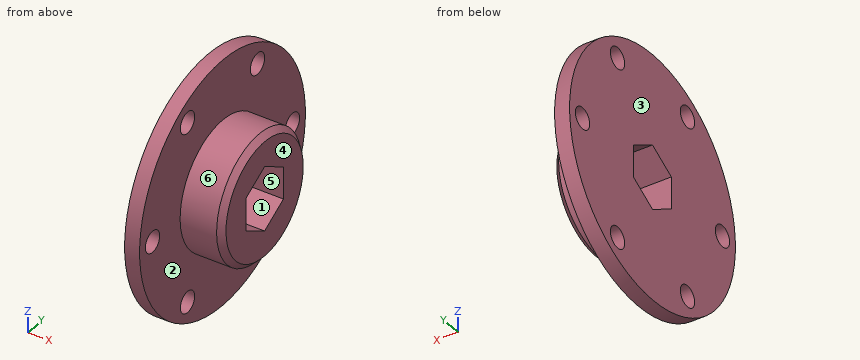
```python
from build123d import *

# Parameters (mm, degrees)
SKETCH1_R           = 27.94
SKETCH1_R_2         = 2.413
BOSS_EXTRUDE1_DEPTH = 3.3909
SKETCH2_R           = 14.2875
BOSS_EXTRUDE2_DEPTH = 9.525
CHAMFER1_SIZE       = 1.27


with BuildPart() as part:
    # Sketch1 → Boss-Extrude1 (new body)
    with BuildSketch(Plane(origin=(0, 0, 0), x_dir=(0, 0, -1), z_dir=(1, 0, 0))):
        Circle(SKETCH1_R)
        with Locations((0, 23.5839)):
            Circle(SKETCH1_R_2, mode=Mode.SUBTRACT)
        with Locations((20.42425652, 11.79195)):
            Circle(SKETCH1_R_2, mode=Mode.SUBTRACT)
        with Locations((20.42425652, -11.79195)):
            Circle(SKETCH1_R_2, mode=Mode.SUBTRACT)
        with Locations((0, -23.5839)):
            Circle(SKETCH1_R_2, mode=Mode.SUBTRACT)
        with Locations((-20.42425652, -11.79195)):
            Circle(SKETCH1_R_2, mode=Mode.SUBTRACT)
        with Locations((-20.42425652, 11.79195)):
            Circle(SKETCH1_R_2, mode=Mode.SUBTRACT)
        Polygon((7.332348419, 0), (3.666174209, 6.35), (-3.666174209, 6.35), (-7.332348419, 0), (-3.666174209, -6.35), (3.666174209, -6.35), align=None, mode=Mode.SUBTRACT)
    extrude(amount=BOSS_EXTRUDE1_DEPTH)

    # Sketch2 → Boss-Extrude2 (add)
    with BuildSketch(Plane(origin=(3.3909, 0, 0), x_dir=(0, 0, -1), z_dir=(1, 0, 0))):
        Circle(SKETCH2_R)
        Polygon((3.666174209, -6.35), (7.332348419, 0), (3.666174209, 6.35), (-3.666174209, 6.35), (-7.332348419, 0), (-3.666174209, -6.35), align=None, mode=Mode.SUBTRACT)
    extrude(amount=BOSS_EXTRUDE2_DEPTH)

    # Chamfer1
    chamfer1_edges = [part.edges().sort_by_distance(p)[0] for p in [
        (12.9159, 0, 14.2875),
    ]]
    chamfer(chamfer1_edges, length=CHAMFER1_SIZE)


solid = part.part
```
Work out the finished part from the listing and answer in its coordinate system (mm). Face numbers are marked on the shaded views. A direction names the side the tool comes from. Coordinates: 2 decimals unless noted, no trailing zeros. Order: outer loops, then holes, each group sorted by start corner. A loop starts at its lowest first (then second) coordinate and runs counter-clockwise, first axis right, second up. Notation, with made-up numbers: (75.5, 56.5) - (114.5, 56.5) arc R30 ccw to (114.5, 88.5) - close; hole circle Ø4 at (27.25, 41.5). An arc over 180 degrees is marked (long way). Answer as a JSON object with one key per item and string values.
1. Consider line 1 (Z direction, x = 2.75, y = -12.5); line 2 (Y direction, x = 3, z = -2); line 3 (X direction, y = 16, z = -7.5). Determine where each line is inside the solid, lowest interval first.
Output values:
{"line 1": "z = -24.99 to -22.73, -18.12 to 18.12, 22.73 to 24.99", "line 2": "y = -27.87 to -24.93, -22.23 to -6.35, 6.35 to 22.23, 24.93 to 27.87", "line 3": "x = 0 to 3.39"}
2. Find section A-A on z = 0. Determine the outline of the cut face in (x, y), plus the area to 3 significant figures.
Output values:
{"outline": "(0, -27.94) - (3.39, -27.94) - (3.39, -26) - (0, -26) - close; (0, -21.17) - (3.39, -21.17) - (3.39, -14.29) - (11.65, -14.29) - (12.92, -13.02) - (12.92, -6.35) - (0, -6.35) - close; (0, 6.35) - (12.92, 6.35) - (12.92, 13.02) - (11.65, 14.29) - (3.39, 14.29) - (3.39, 21.17) - (0, 21.17) - close; (0, 26) - (3.39, 26) - (3.39, 27.94) - (0, 27.94) - close", "area": "263 mm²"}
3. A tool of negligible diameter and unlimited length cuts with its end or side. For the marked faces 1, 2 and 3, from which of +Z, -Z, +X, -X, +Y, -Y can it reach the whole face along a straight path? Write none if from no direction.
Output values:
{"face 1": "+X, -X", "face 2": "+X", "face 3": "+Z, -Z, -X, +Y, -Y"}
4. The mould has two halves that part along Z. Classify the marked faces 4, 5 and 6: +Z half, -Z half, draft (parallel to the pull), parting line (faces both ways), or undercut.
Output values:
{"face 4": "draft", "face 5": "undercut", "face 6": "parting line"}
5. Each of these flat-tipped pins is pushed along its axis until it touches: P1, Ø2, axis at y = 20, z = -5.5, coming from the +X side; P2, Ø3.5, axis at x = 8.5, z = -1, coming from the +Y side; P3, Ø6, axis at x = 10.5, z = -9.5, coming from the +Y side. Where does it stop, or does it pass through?
Output values:
{"P1": "stops at x = 3.39", "P2": "stops at y = 14.29", "P3": "stops at y = 12.72"}
6. Find section C-C on y = 18.5. Determine the outline of the cut face in (x, z), plus the area to 3 significant figures.
Output values:
{"outline": "(0, -20.94) - (3.39, -20.94) - (3.39, 20.94) - (0, 20.94) - close", "area": "142 mm²"}
7. Find section D-D on y = -19. Determine the outline of the cut face in (x, z).
Output values:
{"outline": "(0, -20.49) - (3.39, -20.49) - (3.39, 20.49) - (0, 20.49) - close"}
